Input: part model. Units: mm. Frame: model coordinates. Face numbers are marked on the shaded views. A direction names the side the tool comes from. Give positions to 0.01 mm unless a question says otherwise; leave off trailing zeros. Write each loop counter-clockwise with the first axis right and the second up, starting at its lowest first coordinate (ties: lowest second). Pieces come first, ordered by that corner, then holes. Notation, with made-up numbers: (43.5, -28.75) - (55.5, -28.75) arc R18 cw to (55.5, -18.75) - close; hole circle Ø10 at (-33.5, 15.5). An arc over 180 degrees is marked (long way). Answer as CSV lines item,"result".
```python
from build123d import *
from build123d.topology import SkipClean

# Parameters (mm, degrees)
SKETCH2_R                = 38.1
SKETCH2_R_2              = 35.56
BOSS_EXTRUDE1_DEPTH      = 12.7
SKETCH4_W                = 15.24
SKETCH4_H                = 5.08
BOSS_EXTRUDE2_DEPTH      = 12.7
BOSS_EXTRUDE2_2_DEPTH    = 12.7
SKETCH5_W                = 25.4
SKETCH5_H                = 5.08
BOSS_EXTRUDE4_DEPTH      = 12.7
BOSS_EXTRUDE4_2_DEPTH    = 12.7
BOSS_EXTRUDE5_REACH      = 95.291
BOSS_EXTRUDE5_END_RADIUS = 38.1
SKETCH6_W                = 25.4
SKETCH6_H                = 12.7
BOSS_EXTRUDE6_REACH      = 95.291
BOSS_EXTRUDE6_END_RADIUS = 38.1
SKETCH7_W                = 25.4
SKETCH7_H                = 12.7
SKETCH8_R                = 25.4
BOSS_EXTRUDE7_DEPTH      = 3.81
BOSS_EXTRUDE8_START      = 5.08
SKETCH9_R                = 36.83
SKETCH9_R_2              = 35.56
BOSS_EXTRUDE8_DEPTH      = 5.08
BOSS_EXTRUDE9_START      = 7.62
SKETCH10_R               = 38.1
SKETCH10_R_2             = 35.56
BOSS_EXTRUDE9_DEPTH      = 7.62
SKETCH13_W               = 2.54
SKETCH13_H               = 20.32
CUT_EXTRUDE2_DEPTH       = 98.313021537
CUT_EXTRUDE3_DEPTH       = 123.732886223
CUT_EXTRUDE3_DEPTH_BACK  = 123.732886223
SKETCH14_R               = 4


with BuildPart() as part:
    # Sketch2 → Boss-Extrude1 (new body)
    with BuildSketch(Plane.XY):
        Circle(SKETCH2_R)
        Circle(SKETCH2_R_2, mode=Mode.SUBTRACT)
    extrude(amount=BOSS_EXTRUDE1_DEPTH)



with BuildPart() as body_2:
    # Sketch4 → Boss-Extrude2 (new body)
    with BuildSketch(Plane.XY.offset(12.7)):
        with Locations((19.05, 40.64)):
            Rectangle(SKETCH4_W, SKETCH4_H)
    extrude(amount=BOSS_EXTRUDE2_DEPTH)


with BuildPart() as body_3:
    # Sketch4 → Boss-Extrude2 2 (new body)
    with BuildSketch(Plane.XY.offset(12.7)):
        with Locations((19.05, -40.64)):
            Rectangle(SKETCH4_W, SKETCH4_H)
    extrude(amount=BOSS_EXTRUDE2_2_DEPTH)


with BuildPart() as body_4:
    # Sketch5 → Boss-Extrude4 (new body)
    with BuildSketch(Plane(origin=(0, 0, 12.7), x_dir=(-1, 0, 0), z_dir=(0, 0, -1))):
        with Locations((-19.05, 40.64)):
            Rectangle(SKETCH5_W, SKETCH5_H)
    extrude(amount=BOSS_EXTRUDE4_DEPTH)


with BuildPart() as body_5:
    # Sketch5 → Boss-Extrude4 2 (new body)
    with BuildSketch(Plane(origin=(0, 0, 12.7), x_dir=(-1, 0, 0), z_dir=(0, 0, -1))):
        with Locations((-19.05, -40.64)):
            Rectangle(SKETCH5_W, SKETCH5_H)
    extrude(amount=BOSS_EXTRUDE4_2_DEPTH)


with BuildPart() as part_1:
    add(part.part)

    add(body_3.part)  # Boss-Extrude5 merges body 3

    add(body_5.part)  # Boss-Extrude5 merges body 5
    # Boss-Extrude5: up to this cylinder (the profile starts outside it)
    boss_extrude5_end = Plane(origin=(0, 0, 6.35), z_dir=(0, 0, -1)) * Cylinder(BOSS_EXTRUDE5_END_RADIUS, 267.782, mode=Mode.PRIVATE)
    # Sketch6 → Boss-Extrude5 (add, up to the surface)
    with BuildSketch(Plane(origin=(0, -38.1, 0), x_dir=(1, 0, 0), z_dir=(0, 1, 0)), mode=Mode.PRIVATE) as boss_extrude5_sk1:
        with Locations((19.05, -6.35)):
            Rectangle(SKETCH6_W, SKETCH6_H)
    boss_extrude5_tool1 = extrude(boss_extrude5_sk1.sketch, amount=BOSS_EXTRUDE5_REACH, mode=Mode.PRIVATE) - boss_extrude5_end
    add(boss_extrude5_tool1.solids().sort_by_distance((19.05, -38.1, 6.35))[0])


    add(body_2.part)  # Boss-Extrude6 merges body 2

    add(body_4.part)  # Boss-Extrude6 merges body 4
    # Boss-Extrude6: up to this cylinder (the profile starts outside it)
    boss_extrude6_end = Plane(origin=(0, 0, 6.35), z_dir=(0, 0, -1)) * Cylinder(BOSS_EXTRUDE6_END_RADIUS, 267.782, mode=Mode.PRIVATE)
    # Sketch7 → Boss-Extrude6 (add, up to the surface)
    with BuildSketch(Plane.XZ.offset(-38.1), mode=Mode.PRIVATE) as boss_extrude6_sk1:
        with Locations((19.05, 6.35)):
            Rectangle(SKETCH7_W, SKETCH7_H)
    boss_extrude6_tool1 = extrude(boss_extrude6_sk1.sketch, amount=BOSS_EXTRUDE6_REACH, mode=Mode.PRIVATE) - boss_extrude6_end
    add(boss_extrude6_tool1.solids().sort_by_distance((19.05, 38.1, 6.35))[0])

    # Sketch8 → Boss-Extrude7 (add)
    with BuildSketch(Plane(origin=(0, 43.18, 0), x_dir=(1, 0, 0), z_dir=(0, 1, 0))):
        with Locations((19.05, -49.630055716)):
            Circle(SKETCH8_R)
    boss_extrude7 = extrude(amount=-BOSS_EXTRUDE7_DEPTH)

    # Mirror1: Boss-Extrude7 across plane
    add(boss_extrude7.mirror(Plane.ZX))

    # Sketch9 → Boss-Extrude8 (add)
    with SkipClean():  # the faces are left unmerged after this step: merging them gives an invalid solid
        with BuildSketch(Plane(origin=(0, 0, 0), x_dir=(-1, 0, 0), z_dir=(0, 0, -1)).offset(BOSS_EXTRUDE8_START)):
            with Locations(Location((0, 0, 0), (0, 0, 180))):
                Circle(SKETCH9_R)
            Circle(SKETCH9_R_2, mode=Mode.SUBTRACT)
        extrude(amount=-BOSS_EXTRUDE8_DEPTH)

    # Sketch10 → Boss-Extrude9 (add)
    with SkipClean():  # the faces are left unmerged after this step: merging them gives an invalid solid
        with BuildSketch(Plane(origin=(0, 0, -5.08), x_dir=(-1, 0, 0), z_dir=(0, 0, -1)).offset(BOSS_EXTRUDE9_START)):
            with Locations(Location((0, 0, 0), (0, 0, 180))):
                Circle(SKETCH10_R)
            Circle(SKETCH10_R_2, mode=Mode.SUBTRACT)
        extrude(amount=-BOSS_EXTRUDE9_DEPTH)

    # Sketch13 → Cut-Extrude2 (cut, through all)
    with SkipClean():  # the faces are left unmerged after this step: merging them gives an invalid solid
        with BuildSketch(Plane(origin=(0, 0, 0), x_dir=(0, 0, -1), z_dir=(1, 0, 0))):
            with Locations((1.27, 0)):
                Rectangle(SKETCH13_W, SKETCH13_H)
        extrude(amount=CUT_EXTRUDE2_DEPTH, mode=Mode.SUBTRACT)

    # Sketch14 → Cut-Extrude3 (cut, two sides: drawn at the far end of the back side and taken through both)
    with SkipClean():  # the faces are left unmerged after this step: merging them gives an invalid solid
        with BuildSketch(Plane(origin=(0, 43.18, 0), x_dir=(1, 0, 0), z_dir=(0, 1, 0)).offset(-CUT_EXTRUDE3_DEPTH_BACK)):
            with Locations(Location((19.05, -49.630055716, 0), (0, 0, 270))):
                Circle(SKETCH14_R)
        extrude(amount=CUT_EXTRUDE3_DEPTH + CUT_EXTRUDE3_DEPTH_BACK, mode=Mode.SUBTRACT)


solid = part_1.part
```
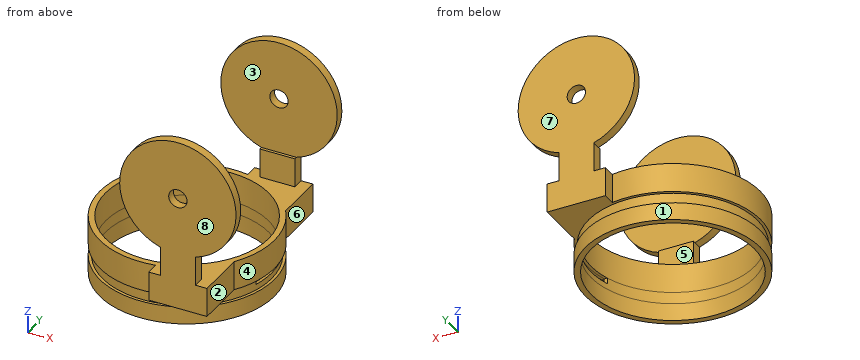
Item 1: Cut plane B-B on x = -4. Return the cut outline in (y, z).
The answers:
outline,"(-43.18, 38.96) - (-39.37, 38.96) - (-39.37, 60.3) - (-43.18, 60.3) - close; (-37.89, -12.7) - (-35.33, -12.7) - (-35.33, 12.7) - (-37.89, 12.7) - (-37.89, 0) - (-36.61, 0) - (-36.61, -5.08) - (-37.89, -5.08) - close; (35.33, -12.7) - (37.89, -12.7) - (37.89, -5.08) - (36.61, -5.08) - (36.61, 0) - (37.89, 0) - (37.89, 12.7) - (35.33, 12.7) - close; (39.37, 38.96) - (43.18, 38.96) - (43.18, 60.3) - (39.37, 60.3) - close"
Item 2: Ray query, line 1 (Y direction, x = 0, z = 6); line 2 (Y direction, x = 0, z = -1); line 3 (Z direction, x = 19.05, y = 40.35). Return the intervals inside material, ascending. Write a range as from..to.
The answers:
line 1,"-38.1..-35.56, 35.56..38.1"
line 2,"-36.83..-35.56, 35.56..36.83"
line 3,"0..45.63, 53.63..75.03"
Item 3: Cut plane D-D on z = 10.5. Return the cut outline in (x, y), plus the area to 3 significant figures.
The answers:
outline,"(6.35, -43.18) - (31.75, -43.18) - (31.75, -21.06) arc R38.1 ccw to (31.75, 21.06) - (31.75, 43.18) - (6.35, 43.18) - (6.35, 37.57) arc R38.1 ccw (long way) to (6.35, -37.57) - close; hole circle Ø71.12 at (0, 0)"
area,"1,160 mm²"
Item 4: Mould query, pull axis Y, two halves, no side actions, for the marked faces 5, 6, 7 and 8. Classes: +Y half, -Y half, draft (parallel to the pull), parting line (faces both ways), or undercut.
The answers:
face 5,"undercut"
face 6,"draft"
face 7,"+Y half"
face 8,"-Y half"
Item 5: Cut plane A-A on y = 0. Return the cut outline in (x, z), plus the area to 3 significant figures.
The answers:
outline,"(-38.1, -12.7) - (-35.56, -12.7) - (-35.56, 12.7) - (-38.1, 12.7) - (-38.1, 0) - (-36.83, 0) - (-36.83, -5.08) - (-38.1, -5.08) - close; (35.56, -12.7) - (38.1, -12.7) - (38.1, -5.08) - (36.83, -5.08) - (36.83, -2.54) - (35.56, -2.54) - close; (35.56, 0) - (38.1, 0) - (38.1, 12.7) - (35.56, 12.7) - close"
area,"113 mm²"
Item 6: Cut plane C-C on y = 12. Return the cut outline in (x, z).
The answers:
outline,"(-36.16, -12.7) - (-33.47, -12.7) - (-33.47, 12.7) - (-36.16, 12.7) - (-36.16, 0) - (-34.82, 0) - (-34.82, -5.08) - (-36.16, -5.08) - close; (33.47, -12.7) - (36.16, -12.7) - (36.16, -5.08) - (34.82, -5.08) - (34.82, 0) - (36.16, 0) - (36.16, 12.7) - (33.47, 12.7) - close"
Item 7: Reachability of the marked faces 1, 2, 3 and 4 from +Z, -Z, +X, -X, +Y, -Y: full face, straight path, thin tool, end or side. Return the list, or none.
The answers:
face 1,"-Z"
face 2,"-Z, +X, -Y"
face 3,"+Z, +X, -X"
face 4,"+Z, -Z, +X"
Item 8: Contact query for flat-ended pins moving along their axis: pin 1 (5.5 mm diameter, centred on y = 40, z = 18, fed in from -X); pin 2 (4 mm diameter, centred on y = -40.5, z = 21, fed in from +X); pin 3 (3 mm diameter, centred on x = 32, z = -2, fed in from -Y); pin 4 (7 mm diameter, centred on x = 19.05, z = 49.63, fed in from -Y). Output: stop coordinate, or through.
The answers:
pin 1,"x = 11.43"
pin 2,"x = 26.67"
pin 3,"y = -20.64"
pin 4,"through"
